```python
from build123d import *

# Parameters (mm, degrees)
SKETCH2_W               = 40
SKETCH2_H               = 48
BOSS_EXTRUDE3_DEPTH     = 3
SKETCH3_W               = 22
SKETCH3_H               = 5
SKETCH3_W_2             = 40
BOSS_EXTRUDE4_DEPTH     = 2.1
SKETCH4_R               = 2.625
CUT_EXTRUDE1_DEPTH      = 1
CUT_EXTRUDE1_DEPTH_BACK = 6.1
SKETCH5_R               = 3.75
CUT_EXTRUDE2_DEPTH      = 3.1
CUT_EXTRUDE2_DEPTH_BACK = 4


with BuildPart() as part:
    # Sketch2 → Boss-Extrude3 (new body)
    with BuildSketch(Plane(origin=(0, 0, 0), x_dir=(1, 0, 0), z_dir=(0, 1, 0))):
        Rectangle(SKETCH2_W, SKETCH2_H)
    extrude(amount=BOSS_EXTRUDE3_DEPTH)

    # Sketch3 → Boss-Extrude4 (add)
    with BuildSketch(Plane(origin=(0, 3, 0), x_dir=(1, 0, 0), z_dir=(0, 1, 0))):
        with Locations((-9, -21.5)):
            Rectangle(SKETCH3_W, SKETCH3_H)
        with BuildLine():
            ThreePointArc((1.125, 0.875), (0.209708691, 3.084708691), (-2, 4))
            Line((-2, 4), (-2, -2.25))
            ThreePointArc((-2, -2.25), (0.209708691, -1.334708691), (1.125, 0.875))
        make_face()
        with BuildLine():
            Line((-2, -2.25), (-2, 4))
            ThreePointArc((-2, 4), (-5.125, 0.875), (-2, -2.25))
        make_face()
        with BuildLine():
            ThreePointArc((10.125, 0.875), (9.209708691, 3.084708691), (7, 4))
            Line((7, 4), (7, -2.25))
            ThreePointArc((7, -2.25), (9.209708691, -1.334708691), (10.125, 0.875))
        make_face()
        with BuildLine():
            Line((7, -2.25), (7, 4))
            ThreePointArc((7, 4), (3.875, 0.875), (7, -2.25))
        make_face()
        with BuildLine():
            Line((7, 4), (-2, 4))
            ThreePointArc((-2, 4), (0.209708691, 3.084708691), (1.125, 0.875))
            ThreePointArc((1.125, 0.875), (0.209708691, -1.334708691), (-2, -2.25))
            Line((-2, -2.25), (7, -2.25))
            ThreePointArc((7, -2.25), (3.875, 0.875), (7, 4))
        make_face()
        with Locations((0, 21.5)):
            Rectangle(SKETCH3_W_2, SKETCH3_H)
    extrude(amount=BOSS_EXTRUDE4_DEPTH)

    # Sketch4 → Cut-Extrude1 (cut, two sides)
    with BuildSketch(Plane(origin=(0, 5.1, 0), x_dir=(1, 0, 0), z_dir=(0, 1, 0))) as cut_extrude1_sk:
        with Locations((2.5, 0.875)):
            Circle(SKETCH4_R)
    extrude(amount=CUT_EXTRUDE1_DEPTH, mode=Mode.SUBTRACT)
    extrude(cut_extrude1_sk.sketch, amount=-CUT_EXTRUDE1_DEPTH_BACK, mode=Mode.SUBTRACT)

    # Sketch5 → Cut-Extrude2 (cut, two sides)
    with BuildSketch(Plane(origin=(0, 3, 0), x_dir=(1, 0, 0), z_dir=(0, 1, 0))) as cut_extrude2_sk:
        with Locations((10, -14)):
            Circle(SKETCH5_R)
    extrude(amount=CUT_EXTRUDE2_DEPTH, mode=Mode.SUBTRACT)
    extrude(cut_extrude2_sk.sketch, amount=-CUT_EXTRUDE2_DEPTH_BACK, mode=Mode.SUBTRACT)


solid = part.part
```
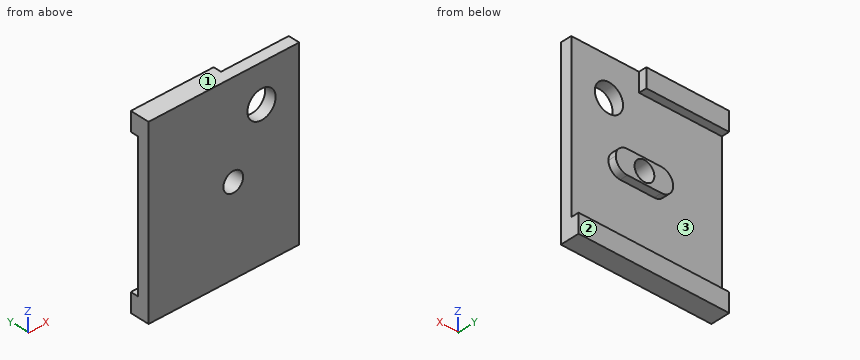
Build history of the part. All positions in model axes, mm. Face numbers are marked on the shaded views. Coordinates: 2 decimals unless noted, no trailing zeros. Order: outer loops, then holes, each group sorted by start corner. A loop starts at its lowest first (then second) coordinate and runs counter-clockwise, first axis right, second up.
Item 1: Drill centre lines: L1, parallel to Z at x = 2.5, y = 3.45; L2, parallel to Z at x = 10, y = 1.55; L3, parallel to X at y = 2.1, z = 14. Where is each one in solid material? Low to high.
Filled in:
L1: z = -24 to -19, -4 to -3.5, 1.75 to 2.25
L2: z = -24 to 10.25, 17.75 to 24
L3: x = -20 to 6.25, 13.75 to 20
Item 2: Mould opens along Z. For the marked faces 1, 2 and 3 say: released by +Z, released by -Z, zero draft, split by the parting line, or undercut.
Filled in:
face 1: released by +Z
face 2: zero draft
face 3: undercut
Item 3: Saw through at C-C on x = -15. List the corners of the cut face in (y, z).
Filled in:
outline: (0, -24) - (5.1, -24) - (5.1, -19) - (3, -19) - (3, 19) - (5.1, 19) - (5.1, 24) - (0, 24) - close
Item 4: Saw through at D-D on z = 7. List the corners of the cut face in (x, y), then the cut area to 3 significant figures.
Filled in:
outline: (-20, 0) - (20, 0) - (20, 3) - (-20, 3) - close
area: 120 mm2
Item 5: Saw through at A-A on z = 17. List the corners of the cut face in (x, y).
Filled in:
outline: (-20, 0) - (7.75, 0) - (7.75, 3) - (-20, 3) - close; (12.25, 0) - (20, 0) - (20, 3) - (12.25, 3) - close
Item 6: Saw through at B-B on y = 3.85. List the corners of the cut face in (x, z) (3 decimals), then the cut area to 3 significant figures.
Filled in:
outline: (-20, -24) - (20, -24) - (20, -19) - (-20, -19) - close; (-20, 19) - (2, 19) - (2, 24) - (-20, 24) - close; (-2, -4) - (7, -4) arc R3.125 ccw to (7, 2.25) - (-2, 2.25) arc R3.125 ccw to start; hole circle Ø5.25 at (2.5, -0.875)
area: 375 mm2
Item 7: Drop flat-ended pins along their axis: pin 1 Ø8 at (x, z) = (-0.5, 13.5) entering from -Y; pin 2 Ø0.6 at (y, z) = (4.5, 22.5) entering from +X. Give the stop position or say it passes through.
Filled in:
pin 1: stops at y = 0
pin 2: stops at x = 2
